```python
from build123d import *

# Parameters (mm, degrees)
SKETCH_1_W          = 22
SKETCH_1_H          = 10
SKETCH_1_R          = 2.5
EXTRUDE_1_DEPTH     = 4
SKETCH_3_R          = 1.75
CUT_EXTRUDE_1_DEPTH = 11
FILLET_1_R          = 2


with BuildPart() as part:
    # ｽｹｯﾁ1 → ﾎﾞｽ - 押し出し1 (new body, symmetric)
    with BuildSketch(Plane.XY):
        Rectangle(SKETCH_1_W, SKETCH_1_H)
        Circle(SKETCH_1_R, mode=Mode.SUBTRACT)
    extrude(amount=EXTRUDE_1_DEPTH, both=True)

    # ｽｹｯﾁ3 → ｶｯﾄ - 押し出し1 (cut, through all)
    with BuildSketch(Plane(origin=(0, 5, 0), x_dir=(1, 0, 0), z_dir=(0, 1, 0))):
        with Locations((7, 0)):
            Circle(SKETCH_3_R)
        with Locations((-7, 0)):
            Circle(SKETCH_3_R)
    extrude(amount=-CUT_EXTRUDE_1_DEPTH, mode=Mode.SUBTRACT)

    # ﾌｨﾚｯﾄ1
    fillet_1_edges = [part.edges().sort_by_distance(p)[0] for p in [
        (-11, 5, 0),
        (11, 5, 0),
    ]]
    fillet(fillet_1_edges, radius=FILLET_1_R)


solid = part.part
```
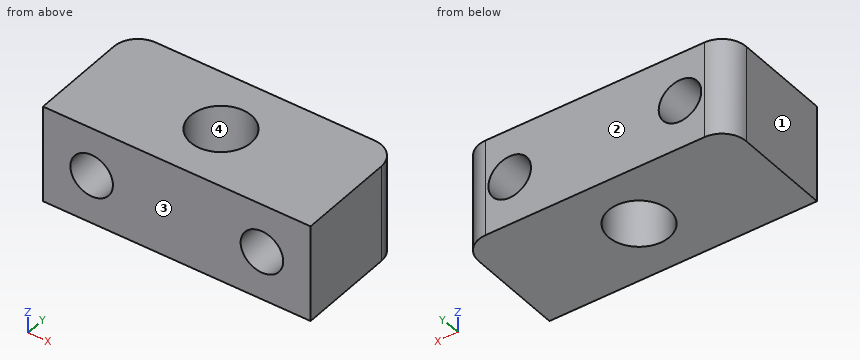
Can you work these out from the model? Positions are in its coordinate system, mm. Face numbers are marked on the shaded views. Round coordinates to 2 decimals unless told otherwise and drop trailing zeros. Loops run counter-clockwise (first coordinate to the right, second up) from the corner with the lowest first, then second, coordinate; pieces in that order, holes last. Notation, with made-up numbers: (59, 7.25) -> (111, 7.25) arc R34 ccw to (111, 37.25) -> close; hole circle Ø8 at (71.25, 61). An arc over 180 degrees is marked (long way). Answer in a Markdown table with one row per item.
Item 1: Suppose I cut it at C-C, the plane z = -3. List the corners of the cut face in (x, y) for me.
Answer block:
| item | result |
|---|---|
| outline | (-11, -5) -> (11, -5) -> (11, 3) arc R2 ccw to (9, 5) -> (-9, 5) arc R2 ccw to (-11, 3) -> close; hole circle Ø5 at (0, 0) |
Item 2: If I drill on probe 1 along Z at (x, y) = (7, 3.25); probe 2 along X at (y, z) = (4.25, -0.25); probe 3 along X at (y, z) = (2.75, 0.25), over which ranges is the centre line in solid material (lowest first)?
Answer block:
| item | result |
|---|---|
| probe 1 | -4 to -1.75, 1.75 to 4 |
| probe 2 | -10.56 to -8.73, -5.27 to 5.27, 8.73 to 10.56 |
| probe 3 | -11 to -8.73, -5.27 to 5.27, 8.73 to 11 |
Item 3: Suppose I cut it at D-D, the plane y = 1.25. List the corners of the cut face in (x, z) for me, plus the area to 3 significant figures.
Answer block:
| item | result |
|---|---|
| outline | (-11, -4) -> (-2.17, -4) -> (-2.17, 4) -> (-11, 4) -> close; (2.17, -4) -> (11, -4) -> (11, 4) -> (2.17, 4) -> close; hole circle Ø3.5 at (-7, 0); hole circle Ø3.5 at (7, 0) |
| area | 122 mm² |
Item 4: Suppose I cut it at A-A, the plane x = 7. List the corners of the cut face in (y, z) for me.
Answer block:
| item | result |
|---|---|
| outline | (-5, -4) -> (5, -4) -> (5, -1.75) -> (-5, -1.75) -> close; (-5, 1.75) -> (5, 1.75) -> (5, 4) -> (-5, 4) -> close |
Item 5: Suppose I cut it at B-B, the plane z = 0. List the corners of the cut face in (x, y) for me.
Answer block:
| item | result |
|---|---|
| outline | (-11, -5) -> (-8.75, -5) -> (-8.75, 5) -> (-9, 5) arc R2 ccw to (-11, 3) -> close; (-5.25, -5) -> (5.25, -5) -> (5.25, 5) -> (-5.25, 5) -> close; (8.75, -5) -> (11, -5) -> (11, 3) arc R2 ccw to (9, 5) -> (8.75, 5) -> close; hole circle Ø5 at (0, 0) |
Item 6: We'd pull the mould along Y, two halves only. Please class the marked faces 1, 2, 3 and 4: released by +Y, released by -Y, zero draft, split by the parting line, or undercut.
Answer block:
| item | result |
|---|---|
| face 1 | zero draft |
| face 2 | released by +Y |
| face 3 | released by -Y |
| face 4 | undercut |
Item 7: Will this pin go through, and if not, where does the flat tip stop? P1, Ø3, axis at x = -0.5, y = 0.5, coming from the +Z side.
Answer block:
| item | result |
|---|---|
| P1 | through |
